The model under review builds one solid part; all positions refer to its coordinate system, in mm. Face numbers are marked on the shaded views. A direction names the side the tool comes from. Round coordinates to 2 decimals unless told otherwise and drop trailing zeros. Loops run counter-clockwise (first coordinate to the right, second up) from the corner with the lowest first, then second, coordinate; pieces in that order, holes last. Notation, with made-up numbers: (50.25, 16.5) -> (63.25, 16.5) arc R17 ccw to (63.25, 38.5) -> close; hole circle Ø5 at (-22.75, 58.25). An arc over 180 degrees is marked (long way). Use a Markdown table: item, result. Add a question column.
1) Insertion check: pin 1 (9.5 mm diameter, centred on x = 8, z = 8.5, fed in from -Y); pin 2 (0.6 mm diameter, centred on x = 54, z = 4.5, fed in from +Y); pin 3 (3 mm diameter, centred on x = 54.5, z = 4.5, fed in from -Y); pin 4 (12 mm diameter, centred on y = 74, z = 2, fed in from +X). Each pin has a flat end and moves straight along its axis. Give the tip position at first contact, or say it passes through.
2) Consider section B-B on y = 66.5. Give the boundary of the cut face in (x, z), plus the area to 3 significant figures.
3) Mouldability with a two-part tool opening along Y and no side actions: class the marked faces 4, 5 and 6 as released by +Y, released by -Y, zero draft, split by the parting line, or undercut.
4) Consider section A-A on x = 137. Give the boundary of the cut face in (y, z), plus the area to 3 significant figures.
5) Wall thickness on probe 1 along Z at (x, y) = (88, 32.5); probe 2 along Y at (x, z) = (12.5, 15); probe 3 along Z at (x, y) = (10.5, 33.5): over which ranges is each line inside the solid? List them lowest first.
6) For the marked faces 1, 2 and 3, list the 3-axis set-ups (+Z, -Z, +X, -X, +Y, -Y) from which the entire face can be reached by the end or side of a thin tool; tool diameter is ignored.
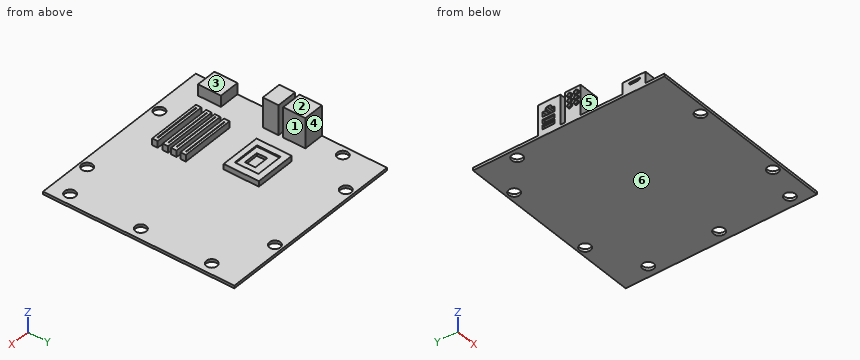
from build123d import *

# Parameters (mm, degrees)
F0_W      = 177.8
F0_H      = 177.8
F1_DEPTH  = 2.54
F2_W      = 19.1831439734
F2_H      = 20.6477418542
F3_DEPTH  = 27.94
F4_W      = 10.8400657773
F4_H      = 3.8665086031
F4_W_2    = 8.9492797852
F4_H_2    = 0.5875341594
F4_H_3    = 4.1402
F4_H_4    = 0.6094495766
F5_DEPTH  = 10.16
F6_W      = 19.1831439734
F6_H      = 14.6254822612
F7_DEPTH  = 27.686
F8_R      = 2.032
F8_R_2    = 1.778
F9_DEPTH  = 1.016
F10_DEPTH = 8.636
F11_W     = 19.1831439734
F11_H     = 21.3800407946
F12_DEPTH = 10.414
F13_W     = 5.7303234935
F13_H     = 0.4988447763
F14_DEPTH = 9.906
F15_R     = 5.08
F16_DEPTH = 2.54
F17_W     = 38.2843576372
F17_H     = 32.6922535896
F17_W_2   = 25.8096791804
F17_H_2   = 21.9382196665
F18_DEPTH = 5.08
F17_W_3   = 13.8996914029
F17_H_3   = 9.7035616636
F19_DEPTH = 3.81
F20_DEPTH = 1.27
F21_W     = 50.8
F21_H     = 5.08
F21_W_2   = 44.6351096034
F21_H_2   = 0.4938840866
F21_H_3   = 0.4938878119
F21_H_4   = 0.7408298552
F22_DEPTH = 6.096


with BuildPart() as f1:
    # F0 (on Top) → F1 (new body)
    with BuildSketch(Plane.XY):
        with Locations((88.9, 88.9)):
            Rectangle(F0_W, F0_H)
    extrude(amount=-F1_DEPTH)

    # F2 (on face) → F3 (join)
    with BuildSketch(Plane.XY):
        with Locations((9.5915719867, 106.9360487163)):
            Rectangle(F2_W, F2_H)
    extrude(amount=F3_DEPTH)

    # F4 (on face) → F5 (cut)
    with BuildSketch(Plane(origin=(0, 0, 0), x_dir=(0, -1, 0), z_dir=(-1, 0, 0))):
        Polygon((-113.1303757429, 19.7547134012), (-113.1303757429, 15.1992412284), (-102.2903099656, 15.1992412284), (-102.2903099656, 19.7547134012), (-104.7438830137, 19.7547134012), (-104.7438830137, 21.687336266), (-106.1243340373, 22.7916929871), (-109.1613098979, 22.7916929871), (-110.4037165642, 21.687336266), (-110.4037165642, 19.7547134012), align=None)
        with Locations((-107.7103428543, 10.8821820468)):
            Rectangle(F4_W, F4_H)
        with Locations((-107.65363276, 11.8099479005)):
            Rectangle(F4_W_2, F4_H_2, mode=Mode.SUBTRACT)
        with Locations((-107.7103428543, 5.8125033508)):
            Rectangle(F4_W, F4_H_3)
        with Locations((-107.65363276, 6.507754093)):
            Rectangle(F4_W_2, F4_H_4, mode=Mode.SUBTRACT)
    extrude(amount=-F5_DEPTH, mode=Mode.SUBTRACT)

    # F6 (on face) → F7 (join)
    with BuildSketch(Plane.XY):
        with Locations((9.5915719867, 84.9978215992)):
            Rectangle(F6_W, F6_H)
    extrude(amount=F7_DEPTH)

    # F8 (on face) → F9 (join)
    with BuildSketch(Plane(origin=(0, 0, 0), x_dir=(0, -1, 0), z_dir=(-1, 0, 0))):
        with Locations((-81.389054656, 22.3253723234)):
            Circle(F8_R)
        with Locations((-81.389054656, 22.3253723234)):
            Circle(F8_R_2, mode=Mode.SUBTRACT)
        with Locations((-87.5466763973, 22.3253723234)):
            Circle(F8_R)
        with Locations((-87.5466763973, 22.3253723234)):
            Circle(F8_R_2, mode=Mode.SUBTRACT)
        with Locations((-81.389054656, 17.514731735)):
            Circle(F8_R)
        with Locations((-81.389054656, 17.514731735)):
            Circle(F8_R_2, mode=Mode.SUBTRACT)
        with Locations((-87.5466763973, 17.514731735)):
            Circle(F8_R)
        with Locations((-87.5466763973, 17.514731735)):
            Circle(F8_R_2, mode=Mode.SUBTRACT)
        with Locations((-87.5466763973, 12.9927285016)):
            Circle(F8_R)
        with Locations((-87.5466763973, 12.9927285016)):
            Circle(F8_R_2, mode=Mode.SUBTRACT)
        with Locations((-81.389054656, 12.9927285016)):
            Circle(F8_R)
        with Locations((-81.389054656, 12.9927285016)):
            Circle(F8_R_2, mode=Mode.SUBTRACT)
    extrude(amount=F9_DEPTH)

    # F10 (cut): faces of the model
    f10_faces = [f1.faces().sort_by_distance(p)[0] for p in [
        (0, 87.5466763973, 22.3253723234),
        (0, 81.389054656, 22.3253723234),
        (0, 81.389054656, 17.514731735),
        (0, 87.5466763973, 17.514731735),
        (0, 87.5466763973, 12.9927285016),
        (0, 81.389054656, 12.9927285016),
    ]]
    extrude(f10_faces, amount=-F10_DEPTH, mode=Mode.SUBTRACT)

    # F11 (on face) → F12 (join)
    with BuildSketch(Plane.XY):
        with Locations((9.5915719867, 28.152519837)):
            Rectangle(F11_W, F11_H)
    extrude(amount=F12_DEPTH)

    # F13 (on face) → F14 (cut)
    with BuildSketch(Plane(origin=(0, 0, 0), x_dir=(0, -1, 0), z_dir=(-1, 0, 0))):
        Polygon((-22.7655656636, 7.4490238912), (-32.3871783912, 7.4490238912), (-32.6265096664, 7.4490238912), (-32.6265096664, 6.2306667678), (-31.4621403813, 5.4544191808), (-24.1432320327, 5.4544191808), (-22.7655656636, 6.1802398413), align=None)
        with Locations((-27.5743678212, 6.5413808916)):
            Rectangle(F13_W, F13_H, mode=Mode.SUBTRACT)
    extrude(amount=-F14_DEPTH, mode=Mode.SUBTRACT)

    # F15 (on face) → F16 (cut)
    with BuildSketch(Plane.XY):
        with Locations((8.3175301552, 143.3550566435)):
            Circle(F15_R)
        with Locations((38.9705635607, 170.5999225378)):
            Circle(F15_R)
        with Locations((121.8317523599, 170.8181649446)):
            Circle(F15_R)
        with Locations((167.6036119461, 148.6765746641)):
            Circle(F15_R)
        with Locations((167.6036119461, 82.7650804687)):
            Circle(F15_R)
        with Locations((167.6036119461, 17.0247107744)):
            Circle(F15_R)
        with Locations((135.1055949926, 6.9549023174)):
            Circle(F15_R)
        with Locations((50.8853644133, 6.9549023174)):
            Circle(F15_R)
    extrude(amount=-F16_DEPTH, mode=Mode.SUBTRACT)

    # F17 (on face) → F18 (join)
    with BuildSketch(Plane.XY):
        with Locations((56.3920978457, 102.6344373822)):
            Rectangle(F17_W, F17_H)
        with Locations((56.1770182103, 102.4193540215)):
            Rectangle(F17_W_2, F17_H_2, mode=Mode.SUBTRACT)
    extrude(amount=F18_DEPTH)

    # F17 (on face) → F19 (join)
    with BuildSketch(Plane.XY):
        with Locations((56.1770182103, 102.4193540215)):
            Rectangle(F17_W_2, F17_H_2)
        with Locations((56.2145523727, 100.97207129)):
            Rectangle(F17_W_3, F17_H_3, mode=Mode.SUBTRACT)
    extrude(amount=F19_DEPTH)

    # F20 (add): a face of the model
    f20_faces = [f1.faces().sort_by_distance(p)[0] for p in [
        (56.2145523727, 100.97207129, 0),
    ]]
    extrude(f20_faces, amount=F20_DEPTH)

    # F21 (on face) → F22 (join)
    with BuildSketch(Plane.XY):
        with Locations((60.0478819847, 56.5112678027)):
            Rectangle(F21_W, F21_H)
        with Locations((59.5629252493, 56.7567013204)):
            Rectangle(F21_W_2, F21_H_2, mode=Mode.SUBTRACT)
        with Locations((60.0478819847, 47.9808410323)):
            Rectangle(F21_W, F21_H)
        with Locations((59.5629252493, 47.9284580797)):
            Rectangle(F21_W_2, F21_H_3, mode=Mode.SUBTRACT)
        with Locations((60.0478819847, 40.0191096282)):
            Rectangle(F21_W, F21_H)
        with Locations((59.5629252493, 40.0879886001)):
            Rectangle(F21_W_2, F21_H_3, mode=Mode.SUBTRACT)
        with Locations((60.0478819847, 30.3512883997)):
            Rectangle(F21_W, F21_H)
        with Locations((59.5629252493, 30.3337052464)):
            Rectangle(F21_W_2, F21_H_4, mode=Mode.SUBTRACT)
    extrude(amount=F22_DEPTH)


solid = f1.part
Result set:
| question | item | result |
|---|---|---|
| 1 | pin 1 | y = 17.46 |
| 1 | pin 2 | y = 118.98 |
| 1 | pin 3 | y = 27.81 |
| 1 | pin 4 | x = 177.8 |
| 2 | outline | (0, -2.54) -> (177.8, -2.54) -> (177.8, 0) -> (0, 0) -> close |
| 2 | area | 452 mm2 |
| 3 | face 4 | released by +Y |
| 3 | face 5 | undercut |
| 3 | face 6 | zero draft |
| 4 | outline | (0, -2.54) -> (2.24, -2.54) -> (2.24, 0) -> (0, 0) -> close; (11.67, -2.54) -> (177.8, -2.54) -> (177.8, 0) -> (11.67, 0) -> close |
| 4 | area | 428 mm2 |
| 5 | probe 1 | -2.54 to 0 |
| 5 | probe 2 | 77.69 to 92.31, 96.61 to 117.26 |
| 5 | probe 3 | -2.54 to 10.41 |
| 6 | face 1 | +Z, +Y, -Y |
| 6 | face 2 | +Z, +X, -X, +Y, -Y |
| 6 | face 3 | +Z, +X, -X, -Y |
